Geometry check sheet. Reference: the model listing, model coordinates, mm. A direction names the side the tool comes from. Coordinates: 2 decimals unless noted, no trailing zeros. Write each loop counter-clockwise with the first axis right and the second up, starting at its lowest first coordinate (ties: lowest second). Pieces come first, ordered by that corner, then holes. Notation, with made-up numbers: (85.25, 29) -> (95.25, 29) arc R12 cw to (95.25, 49) -> close; hole circle Ø9 at (1.5, 18). An arc over 180 degrees is marked (long way). Answer as CSV lines item,"result".
```python
from build123d import *

# Parameters (mm, degrees)
F0_R     = 37.55585
F1_DEPTH = 50.8
F2_W     = 27.772067
F2_H     = 17.381157
F3_DEPTH = 50.8


with BuildPart() as f1:
    # F0 (on Front) → F1 (new body)
    with BuildSketch(Plane.XZ):
        Circle(F0_R)
    extrude(amount=F1_DEPTH)

    # F2 (on Front) → F3 (join)
    with BuildSketch(Plane.XZ):
        with Locations((1.355114, -0.094462)):
            Rectangle(F2_W, F2_H)
    extrude(amount=-F3_DEPTH)


solid = f1.part
```
Item 1: Cross-section at B-B, the plane z = 0. Record the cut outline in (x, y).
Responses:
outline,"(-37.56, -50.8) -> (37.56, -50.8) -> (37.56, 0) -> (15.24, 0) -> (15.24, 50.8) -> (-12.53, 50.8) -> (-12.53, 0) -> (-37.56, 0) -> close"
Item 2: Depth check by flat-ended pin: pin 1 Ø19 at (y, z) = (25.5, 0) entering from -X; pin 2 Ø22 at (x, y) = (-1.5, 28.5) entering from -Z; pin 3 Ø12 at (x, y) = (8, -8.5) entering from -Z; pin 4 Ø10 at (y, z) = (-28, 1.5) entering from +X. Enter the tip coordinate at first touch or a pass-through.
Responses:
pin 1,"stops at x = -12.53"
pin 2,"stops at z = -8.79"
pin 3,"stops at z = -37.5"
pin 4,"stops at x = 37.56"
Item 3: Thickness scan on probe 1 along Y at (x, z) = (-27, 13); probe 2 along Z at (x, y) = (-7.5, 22); probe 3 along X at (y, z) = (-9, -1). Record the ranges inside material, lowest first.
Responses:
probe 1,"y = -50.8 to 0"
probe 2,"z = -8.79 to 8.6"
probe 3,"x = -37.54 to 37.54"
Item 4: Cross-section at A-A, the plane x = 0. Record the cut outline in (y, z), plus the area to 3 significant figures.
Responses:
outline,"(-50.8, -37.56) -> (0, -37.56) -> (0, -8.79) -> (50.8, -8.79) -> (50.8, 8.6) -> (0, 8.6) -> (0, 37.56) -> (-50.8, 37.56) -> close"
area,"4,700 mm2"
Item 5: Cross-section at D-D, the plane x = 30. Record the cut outline in (y, z).
Responses:
outline,"(-50.8, -22.59) -> (0, -22.59) -> (0, 22.59) -> (-50.8, 22.59) -> close"
Item 6: Cross-section at C-C, the plane y = 39. Record the cut outline in (x, z).
Responses:
outline,"(-12.53, -8.79) -> (15.24, -8.79) -> (15.24, 8.6) -> (-12.53, 8.6) -> close"
Item 7: Set-up check for faces 1 (the flat face through (-12.531, 25, 0)), 2 (the flat face through (1, 25, 8.596)), 3 (the flat face through (1, 25, -8.785)), 4 (the flat face through (15.241, 25, 0)): record each of +Z, -Z, +X, -X, +Y, -Y from which the full face is reachable in a straight line by a thin tool's end or side.
Responses:
face 1,"+Z, -Z, -X, +Y"
face 2,"+Z, +X, -X, +Y"
face 3,"-Z, +X, -X, +Y"
face 4,"+Z, -Z, +X, +Y"
